Verification items for the finished model (mm, model axes). A direction names the side the tool comes from. Round coordinates to 2 decimals unless told otherwise and drop trailing zeros. Write each loop counter-clockwise with the first axis right and the second up, starting at its lowest first coordinate (ties: lowest second). Pieces come first, ordered by that corner, then holes. Notation, with made-up numbers: (39.5, 10) - (78.5, 10) arc R31 ccw to (78.5, 46) - close; hole circle Ø8 at (83.5, 78). An arc over 180 degrees is marked (long way). Answer as a JSON object with one key per item and string values.
Autodesk Inventor part; units mm, degrees
ref_plane "YZ Plane" through (0, 0, 0) normal (1, 0, 0) x (0, 1, 0)
ref_plane "XZ Plane" through (0, 0, 0) normal (0, 1, 0) x (-1, 0, 0)
ref_plane "XY Plane" through (0, 0, 0) normal (0, 0, 1) x (1, 0, 0)
sketch "Sketch1" plane through (0, 0, 0) normal (0, 0, 1) x (1, 0, 0)
  line L0 (0, 5.6) -> (0, -5.6)
  line L1 (-5.6, 0) -> (5.6, 0)
  circle A0 centre (0, 0) radius 4
  dimension "d0" = 8
extrude "Extrusion1" add sketch "Sketch1" along normal blind 15
chamfer "Chamfer1" distance 1 angle 45 1 edges at (-4, 0, 0)
chamfer "Chamfer2" distance 0.5 angle 45 1 edges at (-4, 0, 15)
sketch "Sketch2" plane through (0, 0, 15) normal (0, 0, 1) x (1, 0, 0)
  circle A0 centre (0, 0) radius 3.5
  line L0 (2, -1.1547) -> (0, -2.3094)
  line L1 (0, -2.3094) -> (-2, -1.1547)
  line L2 (-2, -1.1547) -> (-2, 1.1547)
  line L3 (-2, 1.1547) -> (0, 2.3094)
  line L4 (0, 2.3094) -> (2, 1.1547)
  line L5 (2, 1.1547) -> (2, -1.1547)
  line L6 (0, 5.6) -> (0, -5.6)
  dimension "d9" = 2
extrude "Extrusion2" cut sketch "Sketch2" against normal blind 3 contours L6 L1 L2 L3 | L4 L5 L0 L6
thread "Thread1"
properties part number "SCREW,SET,CUP POINT,SS, M8X1.25X15MM" material "Stainless Steel, 304L"
1. Go/stop test with flat-tipped pins: pin 1 (4.5 mm diameter, centred on x = 0, y = 0.5, fed in from +Z); pin 2 (1.5 mm diameter, centred on x = -2.5, z = 13, fed in from +Y); pin 3 (2 mm diameter, centred on y = -2, z = 11.5, fed in from -X). Record where each tip stops, or that it passes through.
Completed:
{"pin 1": "stops at z = 15", "pin 2": "stops at y = 3.6", "pin 3": "stops at x = -3.87"}
2. Material ranges on probe 1 along Z at (x, y) = (-1.25, -1); probe 2 along Y at (x, z) = (1.75, 12.75); probe 3 along X at (y, z) = (1, 12.25), recorded low to high. Write a range as from..to.
Completed:
{"probe 1": "z = 0..12", "probe 2": "y = -3.6..-1.3, 1.3..3.6", "probe 3": "x = -3.87..-2, 2..3.87"}
3. Mould release check, pull along Y, two halves, no side actions. Record for faces 1 (the face through (-0.867, 3.905, 7.656)), 2 (the face through (-2, 0, 14)), 3 (the face through (2, -2, 15)): released by +Y, released by -Y, zero draft, split by the parting line, or undercut.
Completed:
{"face 1": "split by the parting line", "face 2": "undercut", "face 3": "zero draft"}
4. Access from +Z, -Z, +X, -X, +Y, -Y to the whole of each face (thin tool, end or side, straight path). Record for faces 4 (the face through (-0.99, -1.74, 13.52)), 5 (the face through (0, 0, 0)).
Completed:
{"face 4": "+Z", "face 5": "-Z, +X, -X, +Y, -Y"}
5. Cross-section at A-A (y = 0). Record the boundary of the cut face in (x, z), plus the area to 3 significant figures.
Completed:
{"outline": "(-4, 1) - (-3, 0) - (3, 0) - (4, 1) - (4, 14.5) - (3.5, 15) - (2, 15) - (2, 12) - (-2, 12) - (-2, 15) - (-3.5, 15) - (-4, 14.5) - close", "area": "107 mm^2"}
6. Cross-section at B-B (z = 6). Record the boundary of the cut face in (x, y), plus the area to 3 significant figures.
Completed:
{"outline": "circle Ø8 at (0, 0)", "area": "50.3 mm^2"}
